CAD build for the part. Positions are in the model's coordinates, mm. Give positions to 0.01 mm unless a question says otherwise; leave off trailing zeros. Write each loop counter-clockwise with the first axis right and the second up, starting at its lowest first coordinate (ties: lowest second). Pieces come first, ordered by that corner, then holes. Notation, with made-up numbers: (3.5, 30.5) - (25.5, 30.5) arc R19 ccw to (25.5, 51.5) - close; hole circle Ø5 at (61.25, 79.25). An arc over 180 degrees is marked (long way). Answer as a JSON object with one key per item and string values.
from build123d import *

# Parameters (mm, degrees)
BOSS_EXTRU_1_DEPTH      = 3
ESQUISSE2_R             = 3.5
ENL_V_MAT_EXTRU_1_DEPTH = 79.04601207


with BuildPart() as part:
    # Esquisse1 → Boss.-Extru.1 (new body)
    with BuildSketch(Plane.XY):
        with BuildLine():
            Line((-55, 20.3), (55, 20.3))
            ThreePointArc((55, 20.3), (75.3, 0), (55, -20.3))
            Line((55, -20.3), (-55, -20.3))
            ThreePointArc((-55, -20.3), (-75.3, 0), (-55, 20.3))
        make_face()
    extrude(amount=BOSS_EXTRU_1_DEPTH)

    # Esquisse2 → Enlèv. mat.-Extru.1 (cut, through all)
    with BuildSketch(Plane.XY.offset(3)):
        with Locations((0, 6)):
            Circle(ESQUISSE2_R)
        with Locations((0, -6)):
            Circle(ESQUISSE2_R)
        with BuildLine():
            Line((-7.5, -8.745966692), (-7.5, 8.745966692))
            ThreePointArc((-7.5, 8.745966692), (-8.057383417, 11.040124031), (-9.605263158, 12.822791267))
            ThreePointArc((-9.605263158, 12.822791267), (-18, 15.5), (-26.394736842, 12.822791267))
            ThreePointArc((-26.394736842, 12.822791267), (-27.942616583, 11.040124031), (-28.5, 8.745966692))
            Line((-28.5, 8.745966692), (-28.5, -8.745966692))
            ThreePointArc((-28.5, -8.745966692), (-27.942616583, -11.040124031), (-26.394736842, -12.822791267))
            ThreePointArc((-26.394736842, -12.822791267), (-18, -15.5), (-9.605263158, -12.822791267))
            ThreePointArc((-9.605263158, -12.822791267), (-8.057383417, -11.040124031), (-7.5, -8.745966692))
        make_face()
        with BuildLine():
            Line((-33.5, -8.745966692), (-33.5, 8.745966692))
            ThreePointArc((-33.5, 8.745966692), (-34.057383417, 11.040124031), (-35.605263158, 12.822791267))
            ThreePointArc((-35.605263158, 12.822791267), (-44, 15.5), (-52.394736842, 12.822791267))
            ThreePointArc((-52.394736842, 12.822791267), (-53.942616583, 11.040124031), (-54.5, 8.745966692))
            Line((-54.5, 8.745966692), (-54.5, -8.745966692))
            ThreePointArc((-54.5, -8.745966692), (-53.942616583, -11.040124031), (-52.394736842, -12.822791267))
            ThreePointArc((-52.394736842, -12.822791267), (-44, -15.5), (-35.605263158, -12.822791267))
            ThreePointArc((-35.605263158, -12.822791267), (-34.057383417, -11.040124031), (-33.5, -8.745966692))
        make_face()
        with BuildLine():
            Line((28.5, 8.745966692), (28.5, -8.745966692))
            ThreePointArc((28.5, -8.745966692), (27.942616583, -11.040124031), (26.394736842, -12.822791267))
            ThreePointArc((26.394736842, -12.822791267), (18, -15.5), (9.605263158, -12.822791267))
            ThreePointArc((9.605263158, -12.822791267), (8.057383417, -11.040124031), (7.5, -8.745966692))
            Line((7.5, -8.745966692), (7.5, 8.745966692))
            ThreePointArc((7.5, 8.745966692), (8.057383417, 11.040124031), (9.605263158, 12.822791267))
            ThreePointArc((9.605263158, 12.822791267), (18, 15.5), (26.394736842, 12.822791267))
            ThreePointArc((26.394736842, 12.822791267), (27.942616583, 11.040124031), (28.5, 8.745966692))
        make_face()
        with BuildLine():
            Line((54.5, 8.745966692), (54.5, -8.745966692))
            ThreePointArc((54.5, -8.745966692), (53.942616583, -11.040124031), (52.394736842, -12.822791267))
            ThreePointArc((52.394736842, -12.822791267), (44, -15.5), (35.605263158, -12.822791267))
            ThreePointArc((35.605263158, -12.822791267), (34.057383417, -11.040124031), (33.5, -8.745966692))
            Line((33.5, -8.745966692), (33.5, 8.745966692))
            ThreePointArc((33.5, 8.745966692), (34.057383417, 11.040124031), (35.605263158, 12.822791267))
            ThreePointArc((35.605263158, 12.822791267), (44, 15.5), (52.394736842, 12.822791267))
            ThreePointArc((52.394736842, 12.822791267), (53.942616583, 11.040124031), (54.5, 8.745966692))
        make_face()
    extrude(amount=-ENL_V_MAT_EXTRU_1_DEPTH, mode=Mode.SUBTRACT)


solid = part.part
(1) Saw through at A-A, the plane x = 0. Give the cut face in (y, z).
Answer key:
{"outline": "(-20.3, 0) - (-9.5, 0) - (-9.5, 3) - (-20.3, 3) - close; (-2.5, 0) - (2.5, 0) - (2.5, 3) - (-2.5, 3) - close; (9.5, 0) - (20.3, 0) - (20.3, 3) - (9.5, 3) - close"}
(2) Saw through at D-D, the plane z = 0.8. State how many separate pieces and enclosed holes the cut face has, and give its area (3 significant figures).
Answer key:
{"separate pieces": "1", "enclosed holes": "6", "area": "3,330 mm²"}
(3) Pull direction X, two halves, no side cores. Call faces 1 (the face through (-53.927, 11.07, 1.521)), 2 (the face through (1, 0, 3)): pulls with the +X half, pulls with the -X half, needs draft (parallel to the pull), parting line crosses it, or undercut.
Answer key:
{"face 1": "undercut", "face 2": "needs draft"}
(4) Flat gauge pins, fed straight in: P1, Ø0.9, axis at y = 3, z = 2, coming from the -X side; P2, Ø0.9, axis at y = -1, z = 1, coming from the -X side; P3, Ø0.9, axis at y = -2.5, z = 2, coming from the +X side. Where does each tip first touch, or does it go through?
Answer key:
{"P1": "stops at x = -75.14", "P2": "stops at x = -75.29", "P3": "stops at x = 75.2"}
(5) Probe L1, parallel to Y at x = 0, z = 1.45; L2, parallel to X at y = -1.5, z = 1; L3, parallel to X at y = 0, z = 0.3. List the from-to ranges inside material, lowest first. Write a range as [from, to].
Answer key:
{"L1": "y = [-20.3, -9.5], [-2.5, 2.5], [9.5, 20.3]", "L2": "x = [-75.24, -54.5], [-33.5, -28.5], [-7.5, 7.5], [28.5, 33.5], [54.5, 75.24]", "L3": "x = [-75.3, -54.5], [-33.5, -28.5], [-7.5, 7.5], [28.5, 33.5], [54.5, 75.3]"}
(6) Saw through at C-C, the plane x = 41. Give the cut face in (y, z), and give its area (3 significant figures).
Answer key:
{"outline": "(-20.3, 0) - (-15.19, 0) - (-15.19, 3) - (-20.3, 3) - close; (15.19, 0) - (20.3, 0) - (20.3, 3) - (15.19, 3) - close", "area": "30.7 mm²"}
(7) Saw through at B-B, the plane y = 0. Give the cut face in (x, z), and give its area (3 significant figures).
Answer key:
{"outline": "(-75.3, 0) - (-54.5, 0) - (-54.5, 3) - (-75.3, 3) - close; (-33.5, 0) - (-28.5, 0) - (-28.5, 3) - (-33.5, 3) - close; (-7.5, 0) - (7.5, 0) - (7.5, 3) - (-7.5, 3) - close; (28.5, 0) - (33.5, 0) - (33.5, 3) - (28.5, 3) - close; (54.5, 0) - (75.3, 0) - (75.3, 3) - (54.5, 3) - close", "area": "200 mm²"}
